from build123d import *

# Parameters (mm, degrees)
F0_W      = 43.5
F0_H      = 3
F1_DEPTH  = 84
F3_DEPTH  = 84
F5_DEPTH  = 43.5
F6_R      = 2
F7_R      = 2
F8_DEPTH  = 4
F9_W      = 1.5
F9_H      = 1.5
F10_DEPTH = 3


# Not quite as in the source:
# - a feature names something its author has since deleted; it is built from what else it names


with BuildPart() as f1:
    # F0 (on Right) → F1 (new body)
    with BuildSketch(Plane.YZ):
        with Locations((21.75, 64.5)):
            Rectangle(F0_W, F0_H)
        Polygon((0, 63), (0, 3), (21, 3), (43.5, 3), (43.5, 63), align=None)
    extrude(amount=-F1_DEPTH)

    # F2 (on Right) → F3 (cut, through all)
    with BuildSketch(Plane.YZ):
        with BuildLine():
            add(Edge.make_bspline(
                [(4.9999998882, 3), (4.9999998882, 32.0000000559), (21.75, 90.0000001676), (38.5000001118, 32.0000000559), (38.5000001118, 3)],
                knots=[0, 0, 0, 0, 0.5, 1, 1, 1, 1], degree=3))
            Line((4.9999998882, 3), (38.5000001118, 3))
        make_face()
    extrude(amount=-F3_DEPTH, mode=Mode.SUBTRACT)

    # F4 (on Front) → F5 (cut, through all)
    with BuildSketch(Plane.XZ):
        with BuildLine():
            add(Edge.make_bspline(
                [(-79.0000001118, 3), (-79.0000001118, 32.0000000559), (-61.7500000559, 90.0000001676), (-44.5, 32.0000000559), (-44.5, 3)],
                knots=[0, 0, 0, 0, 0.5, 1, 1, 1, 1], degree=3))
            Line((-79.0000001118, 3), (-44.5, 3))
        make_face()
        with BuildLine():
            add(Edge.make_bspline(
                [(-39.5, 3), (-39.5, 32.0000000559), (-22.2499999441, 90.0000001676), (-4.9999998882, 32.0000000559), (-4.9999998882, 3)],
                knots=[0, 0, 0, 0, 0.5, 1, 1, 1, 1], degree=3))
            Line((-39.5, 3), (-4.9999998882, 3))
        make_face()
    extrude(amount=-F5_DEPTH, mode=Mode.SUBTRACT)

    # F6
    f6_edges = [f1.edges().sort_by_distance(p)[0] for p in [
        (0, 0, 34.5),
        (-84, 0, 34.5),
        (0, 43.5, 34.5),
        (-84, 43.5, 34.5),
    ]]
    fillet(f6_edges, radius=F6_R)

    # F7 (on face) → F8 (cut)
    with BuildSketch(Plane.XY.offset(66)):
        with Locations((-75, 21.75)):
            Circle(F7_R)
        with Locations((-9, 21.75)):
            Circle(F7_R)
    extrude(amount=-F8_DEPTH, mode=Mode.SUBTRACT)

    # F9 (on face) → F10 (join)
    with BuildSketch(Plane(origin=(0, 0, 3), x_dir=(1, 0, 0), z_dir=(0, 0, -1))):
        with Locations((-42, -2.4999999446)):
            Rectangle(F9_W, F9_H)
        with Locations((-2.4999999441, -2.4999999444)):
            Rectangle(F9_W, F9_H)
        with Locations((-2.4999999443, -41.0000000559)):
            Rectangle(F9_W, F9_H)
        with Locations((-42, -41.0000000564)):
            Rectangle(F9_W, F9_H)
        with Locations((-81.5000000559, -41.0000000561)):
            Rectangle(F9_W, F9_H)
        with Locations((-81.5000000562, -2.4999999441)):
            Rectangle(F9_W, F9_H)
    extrude(amount=F10_DEPTH)


solid = f1.part
For this review, take the finished solid that the model builds, in its own axes (mm). A direction names the side the tool comes from. Give positions to 0.01 mm unless a question says otherwise; leave off trailing zeros.
Item 1: Draft analysis for pull direction Y (two halves, no side actions). For faces 1 (the flat face through (-9, 22, 62)), 2 (the cylindrical face through (-83.43, 42.9, 34.94)), 3 (the flat face through (-39, 0, 43)), state which applies: +Y half, -Y half, draft (parallel to the pull), parting line (faces both ways), or undercut.
Item 2: For line 1 along X through (y, z) = (37.5, 33); line 2 along Y through (x, z) = (-9, 63); line 3 along X through (y, z) = (4.5, 49.5), list the stretches that pass through material, from the lowest coordinate up.
Item 3: Take a section at A-A, the plane z = 33. Give the number of separate pieces and of enclosed holes in the cut face, and give its area (3 significant figures).
Item 4: Insertion check: pin 1 (1.2 mm diameter, centred on x = -81.5, z = 1, fed in from -Y); pin 2 (6 mm diameter, centred on x = -14, z = 44.5, fed in from +Y); pin 3 (1.2 mm diameter, centred on y = 2.5, z = 2, fed in from +X); pin 4 (1.6 mm diameter, centred on y = 2.5, z = 2, fed in from -X). Each pin has a flat end and moves straight along its axis. Give the tip position at first contact, or say it passes through.
Item 5: Tool access review of faces 4 (the cylindrical face through (-73.092, 22.351, 64.028)), 5 (the cylindrical face through (-0.57, 42.9, 34.94)): name each direction out of +Z, -Z, +X, -X, +Y, -Y from which nothing blocks a thin tool from reaching the whole face with its end or side.
Calculated:
1. face 1: undercut
1. face 2: +Y half
1. face 3: -Y half
2. line 1: x = -84 to -76.04, -47.46 to -36.54, -7.96 to 0
2. line 2: y = 0 to 19.75, 23.75 to 43.5
2. line 3: x = -84 to -71.32, -52.18 to -31.82, -12.68 to 0
3. separate pieces: 6
3. enclosed holes: 0
3. area: 419 mm2
4. pin 1: stops at y = 1.75
4. pin 2: stops at y = 43.5
4. pin 3: stops at x = -1.75
4. pin 4: stops at x = -82.25
5. face 4: +Z
5. face 5: +Z, -Z, +X, +Y
